```python
from build123d import *

# Parameters (mm, degrees)
SKETCH1_R           = 9.525
BOSS_EXTRUDE1_DEPTH = 50.8
SKETCH3_R           = 8.509
CUT_EXTRUDE1_DEPTH  = 1.524
SKETCH4_R           = 8.001
CUT_EXTRUDE2_DEPTH  = 50.276


with BuildPart() as part:
    # Sketch1 → Boss-Extrude1 (new body)
    with BuildSketch(Plane(origin=(0, 0, 0), x_dir=(0, 0, -1), z_dir=(1, 0, 0))):
        Circle(SKETCH1_R)
    extrude(amount=BOSS_EXTRUDE1_DEPTH)

    # Sketch3 → Cut-Extrude1 (cut)
    with BuildSketch(Plane.ZY):
        Circle(SKETCH3_R)
    extrude(amount=-CUT_EXTRUDE1_DEPTH, mode=Mode.SUBTRACT)

    # Sketch4 → Cut-Extrude2 (cut, through all)
    with BuildSketch(Plane.ZY.offset(-1.524)):
        Circle(SKETCH4_R)
    extrude(amount=-CUT_EXTRUDE2_DEPTH, mode=Mode.SUBTRACT)


solid = part.part
```
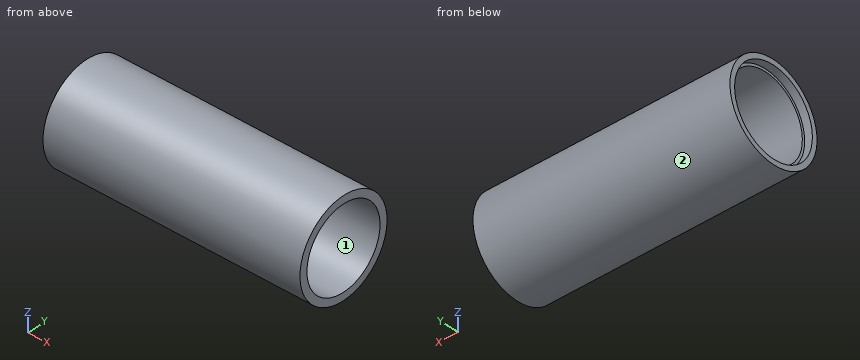
Here's how the part is built. I have some questions about the finished solid (model axes, mm). Face numbers are marked on the shaded views. Give positions to 0.01 mm unless a question says otherwise; leave off trailing zeros. Loops run counter-clockwise (first coordinate to the right, second up) from the corner with the lowest first, then second, coordinate; pieces in that order, holes last. Notation, with made-up numbers: M 69,-30 L 80,-30 A20 cw 80,5 Z; hole C -35.75,-32 d9. An arc over 180 degrees is marked long. Put each result on its own line as item: value. Start each with the question number.
(1) I want a section at A-A on y = 0. Please give me the cut outline in (x, z) (3 decimals).
(2) I want a section at C-C on x = 25. Please give me the cut outline in (y, z) (3 decimals), then the cut area to 3 significant figures.
(3) Will these pins go through, and if not, where does the flat tip stop? pin 1 Ø1 at (x, y) = (27.5, 7) entering from +Z; pin 2 Ø10 at (y, z) = (0.5, 7) entering from -X; pin 3 Ø4 at (x, y) = (7.5, -3.5) entering from -Z.
(4) I need wall thicknesses on line 1 along Y through (x, z) = (1.1, 0) (3 decimals); line 2 along Y through (x, z) = (14.5, 0) (3 decimals); line 3 along X through (y, z) = (1.75, -8). Which ranges of each line are inside material? Lowest first, please. Write a range as [from, to].
(5) If we mould it in two halves opening along Z, with no side actions, what happens to the marked faces 1 and 2? For each: +Z half, -Z half, draft (parallel to the pull), parting line (faces both ways), or undercut.
Answer block:
1. outline: M 0,-9.525 L 50.8,-9.525 L 50.8,-8.001 L 1.524,-8.001 L 1.524,-8.509 L 0,-8.509 Z; M 0,8.509 L 1.524,8.509 L 1.524,8.001 L 50.8,8.001 L 50.8,9.525 L 0,9.525 Z
2. outline: C 0,0 d19.05; hole C 0,0 d16.002
2. area: 83.9 mm^2
3. pin 1: z = 6.96
3. pin 2: x = 0
3. pin 3: z = -9.41
4. line 1: [-9.525, -8.509], [8.509, 9.525]
4. line 2: [-9.525, -8.001], [8.001, 9.525]
4. line 3: [1.52, 50.8]
5. face 1: undercut
5. face 2: parting line
